CAD build for the part. Positions are in the model's coordinates, mm. A direction names the side the tool comes from. Give positions to 0.01 mm unless a question says otherwise; leave off trailing zeros. Write each loop counter-clockwise with the first axis right and the second up, starting at its lowest first coordinate (ties: lowest second). Pieces come first, ordered by that corner, then holes. Notation, with made-up numbers: (56.5, 14.5) - (86.5, 14.5) arc R20 cw to (86.5, 45.5) - close; hole circle Ø1 at (16.25, -17.5). An arc over 180 degrees is marked (long way). Put each result on its own line as item: value. Start each with the question number.
1. Drop flat-ended pins along their axis: pin 1 (15.5 mm diameter, centred on x = -10.5, z = -110, fed in from -Y); pin 2 (10 mm diameter, centred on y = -5, z = -202, fed in from +X); pin 3 (2 mm diameter, centred on x = -7.5, y = -7, fed in from +Z). Give the stop position or say it passes through.
2. Tool access for faces 5 (the flat face through (21, 5, -180)), 6 (the flat face through (0, -6, -174)), 7 (the flat face through (-8, 7, -5)): list every direction of +Z, -Z, +X, -X, +Y, -Y with a clear straight run to the whole face (end or side of a thin tool).
3. Wall check: line 1 (Y direction, x = -7.5, z = -223.25); line 2 (X direction, y = 2, z = -97.5); line 3 (Y direction, x = 6, z = -136). Give the ranges that are in metal, low to high.
4. Mould opens along X. For faces 1 (the cylindrical face through (6.72, -2.8, 13.27)), 2 (the flat face through (0, -7, -200)), 3 (the flat face through (0, 7, 9)), 4 (the cylindrical face through (5.914, 4.93, 9.275)) say: +X half, -X half, draft (parallel to the pull), parting line (faces both ways), or undercut.
5. Cut at B-B on z = -79. List the corners of the cut face in (x, y).
from build123d import *

# Parameters (mm, degrees)
BOSS_EXTRUDE1_DEPTH = 10
SKETCH2_W           = 32
SKETCH2_H           = 15
SKETCH2_R           = 1.75
BOSS_EXTRUDE2_DEPTH = 10
CHAMFER1_SIZE       = 2
SKETCH3_W           = 5
SKETCH3_H           = 5
BOSS_EXTRUDE5_DEPTH = 3
BOSS_EXTRUDE6_START = -5
BOSS_EXTRUDE6_DEPTH = 5
SKETCH7_W           = 2.3
SKETCH7_H           = 1.8
CUT_EXTRUDE2_DEPTH  = 243.991769408
FILLET2_R           = 2
SKETCH8_W           = 10
SKETCH8_H           = 5
BOSS_EXTRUDE7_DEPTH = 10
FILLET3_R           = 10
SKETCH9_W           = 32
SKETCH9_H           = 15
BOSS_EXTRUDE8_DEPTH = 20
FILLET4_R           = 10
CHAMFER2_SIZE       = 12


# Some blends are built 0.0001 mm under size
with BuildPart() as part:
    # Sketch1 → Boss-Extrude1 (new body)
    with BuildSketch(Plane(origin=(0, 0, 0), x_dir=(1, 0, 0), z_dir=(0, 1, 0))):
        with BuildLine():
            ThreePointArc((-16, 0), (0, 16), (16, 0))
            Line((16, 0), (16, 230))
            Line((16, 230), (-16, 230))
            Line((-16, 230), (-16, 0))
        make_face()
        with BuildLine():
            ThreePointArc((-11, 0), (0, 11), (11, 0))
            Line((11, 0), (16, 0))
            ThreePointArc((16, 0), (0, 16), (-16, 0))
            Line((-16, 0), (-11, 0))
        make_face()
        with BuildLine():
            Line((16, 0), (11, 0))
            ThreePointArc((11, 0), (0, -11), (-11, 0))
            Line((-11, 0), (-16, 0))
            ThreePointArc((-16, 0), (0, -16), (16, 0))
        make_face()
    extrude(amount=BOSS_EXTRUDE1_DEPTH)

    # Sketch2 → Boss-Extrude2 (add)
    with BuildSketch(Plane(origin=(0, 0, -230), x_dir=(-1, 0, 0), z_dir=(0, 0, -1))):
        with Locations((0, -7.5)):
            Rectangle(SKETCH2_W, SKETCH2_H)
        with Locations((-7.5, -7)):
            Circle(SKETCH2_R, mode=Mode.SUBTRACT)
        with Locations(Location((7.5, -7, 0), (0, 0, 180))):
            Circle(SKETCH2_R, mode=Mode.SUBTRACT)
    extrude(amount=-BOSS_EXTRUDE2_DEPTH)

    # Chamfer1
    chamfer1_edges = [part.edges().sort_by_distance(p)[0] for p in [
        (0, 0, -220),
    ]]
    chamfer(chamfer1_edges, length=CHAMFER1_SIZE)

    # Sketch3 → Boss-Extrude5 (add)
    with BuildSketch(Plane.XZ.offset(-10)):
        with Locations((0, 8.5)):
            Rectangle(SKETCH3_W, SKETCH3_H)
        Polygon((10.776279442, -3.334936491), (6.446152423, -0.834936491), (3.946152423, -5.165063509), (8.276279442, -7.665063509), align=None)
        Polygon((-8.276279442, -7.665063509), (-3.946152423, -5.165063509), (-6.446152423, -0.834936491), (-10.776279442, -3.334936491), align=None)
    extrude(amount=BOSS_EXTRUDE5_DEPTH)

    # Sketch4 → Boss-Extrude6 (add)
    with BuildSketch(Plane(origin=(0, 0, 0), x_dir=(1, 0, 0), z_dir=(0, 1, 0)).offset(BOSS_EXTRUDE6_START)):
        with BuildLine():
            Line((5, -12), (-5, -12))
            Line((-5, -12), (-5, -15.198684154))
            ThreePointArc((-5, -15.198684154), (0, -16), (5, -15.198684154))
            Line((5, -15.198684154), (5, -12))
        make_face()
    extrude(amount=BOSS_EXTRUDE6_DEPTH)

    # Sketch7 → Cut-Extrude2 (cut, through all)
    with BuildSketch(Plane(origin=(0, 0, 12), x_dir=(-1, 0, 0), z_dir=(0, 0, -1))):
        with Locations((0, -0.9)):
            Rectangle(SKETCH7_W, SKETCH7_H)
    extrude(amount=-CUT_EXTRUDE2_DEPTH, mode=Mode.SUBTRACT)

    # Fillet2
    fillet2_edges = [part.edges().sort_by_distance(p)[0] for p in [
        (2.5, 8.5, 10.712142643),
        (-2.5, 8.5, 10.712142643),
        (8.026987658, 8.5, -7.521134831),
        (10.526987658, 8.5, -3.191007812),
        (-10.526987658, 8.5, -3.191007812),
        (-8.026987658, 8.5, -7.521134831),
    ]]
    fillet(fillet2_edges, radius=FILLET2_R - 0.0001)  # a hair under: the kernel refuses the full size

    # Sketch8 → Boss-Extrude7 (add)
    with BuildSketch(Plane.XZ):
        with Locations((21, -177.5)):
            Rectangle(SKETCH8_W, SKETCH8_H)
        with Locations((-21, -177.5)):
            Rectangle(SKETCH8_W, SKETCH8_H)
    extrude(amount=-BOSS_EXTRUDE7_DEPTH)

    # Fillet3
    fillet3_edges = [part.edges().sort_by_distance(p)[0] for p in [
        (16, 5, -175),
        (-16, 5, -175),
    ]]
    fillet(fillet3_edges, radius=FILLET3_R - 0.0001)  # a hair under: the kernel refuses the full size

    # Sketch9 → Boss-Extrude8 (add)
    with BuildSketch(Plane(origin=(0, 0, -180), x_dir=(-1, 0, 0), z_dir=(0, 0, -1))):
        with Locations((0, -7.5)):
            Rectangle(SKETCH9_W, SKETCH9_H)
    extrude(amount=BOSS_EXTRUDE8_DEPTH)

    # Fillet4
    # the kernel refuses this fillet: 10 mm, written as the material it adds along each edge
    with BuildSketch(Plane(origin=(-5, 0, 12), x_dir=(-1, 0, 0), z_dir=(0, 0, 1))) as fillet4_piece_1_section:
        with BuildLine():
            CenterArc((8.660254038, 10), FILLET4_R, 210, 60)
            Line((0, 5), (0, 0))
            Line((0, 0), (8.660254038, 0))
        make_face()
    fillet4_piece_1 = extrude(amount=24.849319248, mode=Mode.PRIVATE)
    fillet4_piece_1 = fillet4_piece_1 & Plane(origin=(0, 0, 0), x_dir=(-1, 0, 0), z_dir=(0, -1, 0)) * Cylinder(16, 85, mode=Mode.PRIVATE)
    add(fillet4_piece_1)
    with BuildSketch(Plane(origin=(5, 0, 36.849319248), x_dir=(1, 0, 0), z_dir=(0, 0, -1))) as fillet4_piece_2_section:
        with BuildLine():
            CenterArc((8.660254038, 10), FILLET4_R, 210, 60)
            Line((0, 5), (0, 0))
            Line((0, 0), (8.660254038, 0))
        make_face()
    fillet4_piece_2 = extrude(amount=24.849319248, mode=Mode.PRIVATE)
    fillet4_piece_2 = fillet4_piece_2 & Plane(origin=(0, 0, 0), x_dir=(-1, 0, 0), z_dir=(0, -1, 0)) * Cylinder(16, 85, mode=Mode.PRIVATE)
    add(fillet4_piece_2)

    # Chamfer2
    chamfer2_edges = [part.edges().sort_by_distance(p)[0] for p in [
        (0, 0, -180),
    ]]
    chamfer(chamfer2_edges, length=CHAMFER2_SIZE)


solid = part.part
Report:
1. pin 1: stops at y = 0
1. pin 2: stops at x = 16
1. pin 3: stops at z = -174
2. face 5: -Z, +X, +Y, -Y
2. face 6: +X, -X, -Y
2. face 7: -Y
3. line 1: y = -15 to -8.75, -5.25 to 10
3. line 2: x = -16 to 16
3. line 3: y = 0 to 10
4. face 1: +X half
4. face 2: draft
4. face 3: undercut
4. face 4: undercut
5. outline: (-16, 0) - (16, 0) - (16, 10) - (-16, 10) - close
